The drawing under review shows one solid part. Ordinate dimensions are in mm from its lowest x, y, z. A direction names the side the tool comes from. Coordinates: 2 decimals unless noted, no trailing zeros. Write each loop counter-clockwise with the first axis right and the second up, starting at its lowest first coordinate (ties: lowest second). Pieces come first, ordered by that corner, then holes. Notation, with made-up numbers: M 29.25,29 L 88.25,29 A27 ccw 88.25,55 Z; hole C 65,27 d8. An arc over 180 degrees is marked long. Write each question's results on one line, items separated by ' | '. Start each with the question number.
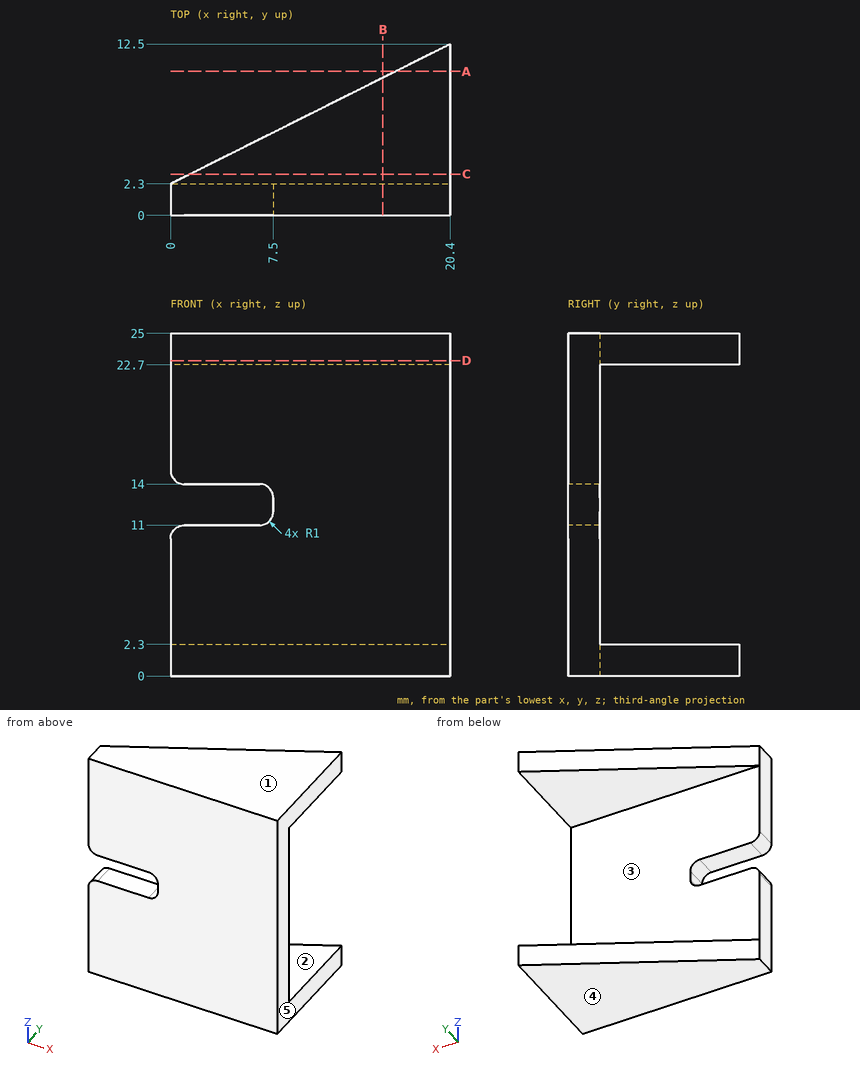
Item 1: We need section A-A on y = 10.5. State the section outline as (x, z) points.
Item 2: Insertion check: pin 1 Ø6 at (x, z) = (7, 8.5) entering from +Y; pin 2 Ø0.8 at (y, z) = (0.5, 12.5) entering from -X; pin 3 Ø3 at (y, z) = (2.5, 13) entering from -X; pin 4 Ø2 at (x, z) = (4, 12.5) entering from -Y. Each pin has a flat end and moves straight along its axis. Give the tip position at first contact, or say it passes through.
Item 3: We need section B-B on x = 15.5. State the section outline as (y, z) points, then the cut area to 4 significant figures.
Item 4: We need section D-D on z = 23. State the section outline as (x, y) points, then the cut area to 3 significant figures.
Item 5: Draft analysis for pull direction Z (two halves, no side actions). For the marked faces 3, 4 and 5, state which applies: released by +Z, released by -Z, zero draft, split by the parting line, or undercut.
Item 6: For the marked faces 1 and 2, list the 3-axis set-ups (+Z, -Z, +X, -X, +Y, -Y) from which the entire face can be reached by the end or side of a thin tool; tool diameter is ignored.
Item 7: We need section C-C on y = 3. State the section outline as (x, z) points.
Item 8: Wall thickness on L1, parallel to Z at x = 17, y = 8; L2, parallel to Y at x = 15, z = 8.75; L3, parallel to Y at x = 6.25, z = 1.75 (3 decimals): over which ranges is each line inside the solid? List them lowest first.
Answer:
1) outline: M 16.4,0 L 20.4,0 L 20.4,2.3 L 16.4,2.3 Z; M 16.4,22.7 L 20.4,22.7 L 20.4,25 L 16.4,25 Z
2) pin 1: stops at y = 2.3 | pin 2: stops at x = 7.5 | pin 3: stops at x = 0.14 | pin 4: passes through
3) outline: M 0,0 L 10.05,0 L 10.05,2.3 L 2.3,2.3 L 2.3,22.7 L 10.05,22.7 L 10.05,25 L 0,25 Z | area: 93.15 mm^2
4) outline: M 0,0 L 20.4,0 L 20.4,12.5 L 0,2.3 Z | area: 151 mm^2
5) face 3: undercut | face 4: released by -Z | face 5: zero draft
6) face 1: +Z, +X, -X, +Y, -Y | face 2: +X, -X, +Y
7) outline: M 1.4,0 L 20.4,0 L 20.4,2.3 L 1.4,2.3 Z; M 1.4,22.7 L 20.4,22.7 L 20.4,25 L 1.4,25 Z
8) L1: z = 0 to 2.3, 22.7 to 25 | L2: y = 0 to 2.3 | L3: y = 0 to 5.425
